The listing builds one solid part. Answer for the finished solid, in the listing's coordinates (mm). A direction names the side the tool comes from. Give positions to 0.01 mm unless a question says otherwise; leave off trailing zeros. Order: outer loops, then holes, each group sorted by start corner. A loop starts at its lowest first (then second) coordinate and runs counter-clockwise, first axis right, second up. Notation, with made-up numbers: (67.5, -20) - (100.5, -20) arc R25 ccw to (100.5, -2) - close; hole circle Ø6 at (58.25, 5.25). An arc over 180 degrees is marked (long way). Answer as CSV lines item,"result". Start each with the question number.
1. Section C-C on z = 2.75 is taken. Count the separate pieces of the cut face and the enclosed holes in it, and give its area (3 significant figures).
2. Section B-B on x = -63.5 is taken. Give the vertices of the cut face in (y, z).
3. Which of the six approach directions +Z, -Z, +X, -X, +Y, -Y give full straight-line access (tool end or side, diameter ignored) to faces 5 (the flat face through (-131.98, -41.76, 2.96)), 6 (the cylindrical face through (-88.74, -151.75, 3.04))?
4. Consider line 1 along Y through (x, z) = (30, 1.5); line 2 along Y through (x, z) = (-71, 2); line 3 along X through (y, z) = (-100, 3.85). Determine where each line is inside the solid, lowest interval first. Write a range as [from, to].
5. Determine the mould class of faces 1 (the cylindrical face through (-78.34, 114.14, 3.04)), 2 (the cylindrical face through (75.634, -163.343, 3.042)), 3 (the cylindrical face through (-115.634, -163.343, 3.042)), 4 (the flat face through (14, -18, 0)) for opening direction X: +X half, -X half, draft (parallel to the pull), parting line (faces both ways), or undercut.
6. Section A-A on y = -85.5 is taken. Give the vertices of the cut face in (x, z), and give its area (3 significant figures).
7. Section D-D on x = -21 is taken. Give the vertices of the cut face in (y, z), and give its area (3 significant figures).
8. Flat-ended cylindrical pins translate along their axes: pin 1 (3 mm diameter, centred on x = 55, y = -104.1, fed in from -Z); pin 2 (1.8 mm diameter, centred on x = 84.5, z = 4, fed in from -Y); pin 3 (3 mm diameter, centred on x = 107.5, z = 2, fed in from +Y); pin 4 (1.8 mm diameter, centred on y = -103, z = 3, fed in from -X). Find the tip coordinate at first contact, or state that the pin passes through.
from build123d import *

# Parameters (mm, degrees)
ESBO_O1_R                = 1.75
ESBO_O1_W                = 30
ESBO_O1_H                = 6.2
ESBO_O1_W_2              = 6.2
ESBO_O1_H_2              = 30
RESSALTO_EXTRUS_O1_DEPTH = 6
FILETE1_R                = 54
FILETE2_R                = 50
ESBO_O2_W                = 14.9
ESBO_O2_H                = 6
CORTE_EXTRUS_O1_DEPTH    = 6.25
ESBO_O3_W                = 1.5
ESBO_O3_H                = 15
CORTE_EXTRUS_O2_DEPTH    = 10
FILETE3_R                = 0.75
CORTE_EXTRUS_O3_DEPTH    = 22


with BuildPart() as part:
    # Esboço1 → Ressalto-extrusão1 (new body)
    with BuildSketch(Plane.XY):
        Polygon((125, -165), (75, -165), (49.019237886, -150), (-89.019237886, -150), (-115, -165), (-165, -165), (-87.294734195, 125), (125, 125), align=None)
        with Locations((-87.583302492, -104.1)):
            Circle(ESBO_O1_R, mode=Mode.SUBTRACT)
        with Locations((120.9, 45)):
            Circle(ESBO_O1_R, mode=Mode.SUBTRACT)
        with Locations((55, -104.1)):
            Circle(ESBO_O1_R, mode=Mode.SUBTRACT)
        with Locations((120.9, -100)):
            Circle(ESBO_O1_R, mode=Mode.SUBTRACT)
        with Locations((80, -104.1)):
            Rectangle(ESBO_O1_W, ESBO_O1_H, mode=Mode.SUBTRACT)
        with Locations((30, -104.1)):
            Rectangle(ESBO_O1_W, ESBO_O1_H, mode=Mode.SUBTRACT)
        with Locations((-112.583302492, -104.1)):
            Rectangle(ESBO_O1_W, ESBO_O1_H, mode=Mode.SUBTRACT)
        with Locations((-62.583302492, -104.1)):
            Rectangle(ESBO_O1_W, ESBO_O1_H, mode=Mode.SUBTRACT)
        with Locations((120.9, 70)):
            Rectangle(ESBO_O1_W_2, ESBO_O1_H_2, mode=Mode.SUBTRACT)
        with Locations((120.9, 20)):
            Rectangle(ESBO_O1_W_2, ESBO_O1_H_2, mode=Mode.SUBTRACT)
        with Locations((120.9, -125)):
            Rectangle(ESBO_O1_W_2, ESBO_O1_H_2, mode=Mode.SUBTRACT)
        with Locations((120.9, -75)):
            Rectangle(ESBO_O1_W_2, ESBO_O1_H_2, mode=Mode.SUBTRACT)
    extrude(amount=RESSALTO_EXTRUS_O1_DEPTH)

    # Filete1
    filete1_edges = [part.edges().sort_by_distance(p)[0] for p in [
        (-87.294734195, 125, 3),
    ]]
    fillet(filete1_edges, radius=FILETE1_R)

    # Filete2
    filete2_edges = [part.edges().sort_by_distance(p)[0] for p in [
        (75, -165, 3),
        (49.019237886, -150, 3),
        (-89.019237886, -150, 3),
        (-115, -165, 3),
    ]]
    fillet(filete2_edges, radius=FILETE2_R)

    # Esboço2 → Corte-extrusão1 (cut)
    with BuildSketch(Plane(origin=(0, 125, 0), x_dir=(1, 0, 0), z_dir=(0, 1, 0))):
        with Locations((110.55, -3)):
            Rectangle(ESBO_O2_W, ESBO_O2_H)
    extrude(amount=-CORTE_EXTRUS_O1_DEPTH, mode=Mode.SUBTRACT)

    # Esboço3 → Corte-extrusão2 (cut)
    with BuildSketch(Plane.XY.offset(6)):
        with Locations((110.55, 111.25)):
            Rectangle(ESBO_O3_W, ESBO_O3_H)
    extrude(amount=-CORTE_EXTRUS_O2_DEPTH, mode=Mode.SUBTRACT)

    # Filete3
    filete3_edges = [part.edges().sort_by_distance(p)[0] for p in [
        (111.3, 103.75, 3),
        (109.8, 103.75, 3),
    ]]
    fillet(filete3_edges, radius=FILETE3_R - 0.0001)  # a hair under: the kernel refuses the full size

    # Esboço4 → Corte-extrusão3 (cut)
    with BuildSketch(Plane.XY.offset(6)):
        Polygon((-149.813874716, -112.188312175), (-153.696160392, -126.677199569), (-150.677642185, -127.486009085), (-146.795356509, -112.997121691), align=None)
        Polygon((-146.795356509, -112.997121691), (-150.677642185, -127.486009085), (-147.659123978, -128.294818601), (-143.776838302, -113.805931207), align=None)
        with BuildLine():
            ThreePointArc((-152.367408211, -133.792301745), (-154.204525518, -134.852961916), (-153.143865346, -136.690079223))
            Line((-153.143865346, -136.690079223), (-152.367408211, -133.792301745))
        make_face()
        with BuildLine():
            Line((-152.367408211, -133.792301745), (-153.143865346, -136.690079223))
            ThreePointArc((-153.143865346, -136.690079223), (-151.842494635, -136.431220494), (-151.255636778, -135.241190484))
            ThreePointArc((-151.255636778, -135.241190484), (-151.565606768, -134.328048341), (-152.367408211, -133.792301745))
        make_face()
        Polygon((-157.578446069, -141.166086963), (-161.460731746, -155.654974358), (-158.442213538, -156.463783874), (-154.559927862, -141.974896479), align=None)
        Polygon((-154.559927862, -141.974896479), (-158.442213538, -156.463783874), (-155.423695331, -157.27259339), (-151.541409655, -142.783705995), align=None)
    extrude(amount=-CORTE_EXTRUS_O3_DEPTH, mode=Mode.SUBTRACT)


solid = part.part
Checks:
1,separate pieces,"1"
1,enclosed holes,"15"
1,area,"68,200 mm²"
2,outline,"(-150, 0) - (-107.2, 0) - (-107.2, 6) - (-150, 6) - close; (-101, 0) - (122.04, 0) - (122.04, 6) - (-101, 6) - close"
3,face 5,"+Z, -Z, -X, +Y"
3,face 6,"+Z, -Z, -Y"
4,line 1,"y = [-150, -107.2], [-101, 125]"
4,line 2,"y = [-150, -107.2], [-101, 118.79]"
4,line 3,"x = [-147.58, 119.15], [122.65, 125]"
5,face 1,"-X half"
5,face 2,"undercut"
5,face 3,"undercut"
5,face 4,"draft"
6,outline,"(-143.7, 0) - (117.8, 0) - (117.8, 6) - (-143.7, 6) - close; (124, 0) - (125, 0) - (125, 6) - (124, 6) - close"
6,area,"1,570 mm²"
7,outline,"(-150, 0) - (125, 0) - (125, 6) - (-150, 6) - close"
7,area,"1,650 mm²"
8,pin 1,"passes through"
8,pin 2,"stops at y = -164.91"
8,pin 3,"stops at y = 118.75"
8,pin 4,"stops at x = -148.63"
